Design review of the part built by this model. Coordinates are the model's own, in mm. Give positions to 0.01 mm unless a question says otherwise; leave off trailing zeros. Loops run counter-clockwise (first coordinate to the right, second up) from the corner with the lowest first, then second, coordinate; pieces in that order, holes last.
from build123d import *

# Parameters (mm, degrees)
F0_W     = 180
F0_H     = 250
F1_DEPTH = 12
F2_W     = 180
F2_H     = 80
F3_DEPTH = 12


with BuildPart() as f1:
    # F0 (on Front) → F1 (new body)
    with BuildSketch(Plane.XZ):
        with Locations((32.637028, -69.309338)):
            Rectangle(F0_W, F0_H)
    extrude(amount=-F1_DEPTH)

    # F2 (on face) → F3 (join)
    with BuildSketch(Plane.XZ):
        with Locations((-57.362972, 95.690662)):
            Rectangle(F2_W, F2_H)
    extrude(amount=-F3_DEPTH)


solid = f1.part
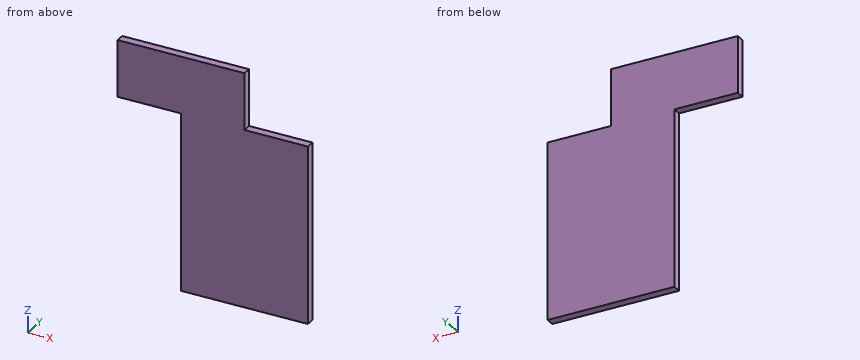
Q1. Insertion check: pin 1 (6 mm diameter, centred on y = 3.5, z = -121.5, fed in from -X); pin 2 (3.5 mm diameter, centred on y = 8.5, z = 101, fed in from +X). Each pin has a flat end and moves straight along its axis. Give the tip position at first contact, or say it passes through.
Results:
pin 1: stops at x = -57.36
pin 2: stops at x = 32.64
Q2. Take a section at C-C (x = -90.5). Give the boundary of the cut face in (y, z), plus the area to 3 significant figures.
Results:
outline: (0, 55.69) - (12, 55.69) - (12, 135.69) - (0, 135.69) - close
area: 960 mm2
Q3. Take a section at B-B (z = -171). Give the boundary of the cut face in (x, y), plus the area to 3 significant figures.
Results:
outline: (-57.36, 0) - (122.64, 0) - (122.64, 12) - (-57.36, 12) - close
area: 2,160 mm2
Q4. Wall thickness on line 1 (Z direction, x = -125.5, y = 6.5); line 2 (Z direction, x = 67, y = 11.75); line 3 (X direction, y = 6.5, z = 71.5): over which ranges is each line inside the solid? List them lowest first.
Results:
line 1: z = 55.69 to 135.69
line 2: z = -194.31 to 55.69
line 3: x = -147.36 to 32.64
Q5. Take a section at A-A (y = 3.75). Give the boundary of the cut face in (x, z).
Results:
outline: (-147.36, 55.69) - (-57.36, 55.69) - (-57.36, -194.31) - (122.64, -194.31) - (122.64, 55.69) - (32.64, 55.69) - (32.64, 135.69) - (-147.36, 135.69) - close
